Here's how the part is built. I have some questions about the finished solid (model axes, mm). Face numbers are marked on the shaded views. A direction names the side the tool comes from. Give positions to 0.01 mm unless a question says otherwise; leave off trailing zeros. Loops run counter-clockwise (first coordinate to the right, second up) from the corner with the lowest first, then second, coordinate; pieces in that order, holes last. Notation, with made-up numbers: (39.5, 20) - (56.5, 20) arc R35 ccw to (56.5, 52) - close; hole circle Ø10 at (3, 20). An arc over 180 degrees is marked (long way). Return JSON: item names as keys, results as strings. Group by question number.
(1) If we section it at A-A (x = 0): Please give me the cut outline in (y, z).
(2) If we section it at D-D (z = 157.5): Please give me the cut outline in (x, y).
(3) I need wall thicknesses on probe 1 along Z at (x, y) = (-4.5, -63); probe 2 along Z at (x, y) = (63.5, 8); probe 3 along Y at (x, z) = (-11, 166). Which ranges of each line are inside material? Lowest first, please. Write a range as [from, to].
(4) If we section it at C-C (x = 49): Please give me the cut outline in (y, z).
(5) For P1, Ø2, axis at y = -14, z = 185, coming from the -X side; P2, Ø22.5, axis at x = 12, z = 157.5, coming from the +Y side; P3, Ø9.5, axis at x = -2, z = 191, coming from the -Y side, each with a flat end and sliding along its axis, tell me the tip position at first contact or that it passes through.
(6) If we mould it in two halves opening along Y, with no side actions, what happens to the marked faces 1, 2 and 3? For each: released by +Y, released by -Y, zero draft, split by the parting line, or undercut.
(7) On a 3-axis mill with a long thin cutter (end or side, diameter ignored), from which of +Z, -Z, +X, -X, +Y, -Y can I reach the whole of each face in a straight line? I mean the marked faces 4 and 5. Say none if no direction works.
(8) If we section it at B-B (y = 0): Please give me the cut outline in (x, z).
Autodesk Inventor part; units mm, degrees
ref_plane "YZ Plane" through (0, 0, 0) normal (1, 0, 0) x (0, 1, 0)
ref_plane "XZ Plane" through (0, 0, 0) normal (0, 1, 0) x (-1, 0, 0)
ref_plane "XY Plane" through (0, 0, 0) normal (0, 0, 1) x (1, 0, 0)
sketch "Sketch1" plane through (0, 0, 0) normal (0, 0, 1) x (1, 0, 0)
  circle A0 centre (0, 0) radius 84
  dimension "d0" = 168
extrude "Extrusion1" add sketch "Sketch1" along normal blind 176
sketch "Sketch2" plane through (0, 0, 0) normal (0, 1, 0) x (-1, 0, 0)
  line L0 (84, 176) -> (-84, 176)
  circle A0 centre (0, 176) radius 28
  point P0 (0, 0)
  dimension "d3" = 56
extrude "Extrusion2" cut sketch "Sketch2" along normal mid plane 120
sketch "Sketch4" plane through (0, 0, 176) normal (0, 0, 1) x (1, 0, 0)
  line L0 (68, -28) -> (-68, -28)
  line L1 (-68, -28) -> (-68, 28)
  line L2 (-68, 28) -> (68, 28)
  line L3 (68, 28) -> (68, -28)
  line L4 (68, -28) -> (-68, 28) construction
  line L5 (-68, -28) -> (68, 28) construction
  circle A0 centre (0, 0) radius 84
  dimension "d7" = 56
  dimension "d8" = 16
extrude "Extrusion3" add sketch "Sketch4" along normal blind 24 contours L0 L1 L2 L3
sketch "Sketch5" plane through (0, 0, 200) normal (0, 0, 1) x (1, 0, 0)
  line L0 (28, -28) -> (-28, -28)
  line L1 (-12, 28) -> (12, 28)
  line L2 (12, 28) -> (12, -28)
  line L3 (12, -28) -> (-12, -28)
  line L4 (-12, -28) -> (-12, 28)
  line L5 (-12, 28) -> (12, -28) construction
  line L6 (12, 28) -> (-12, -28) construction
  point P0 (0, 0)
  dimension "d11" = 24
extrude "Extrusion4" add sketch "Sketch5" along normal blind 8
properties part number "link_1"
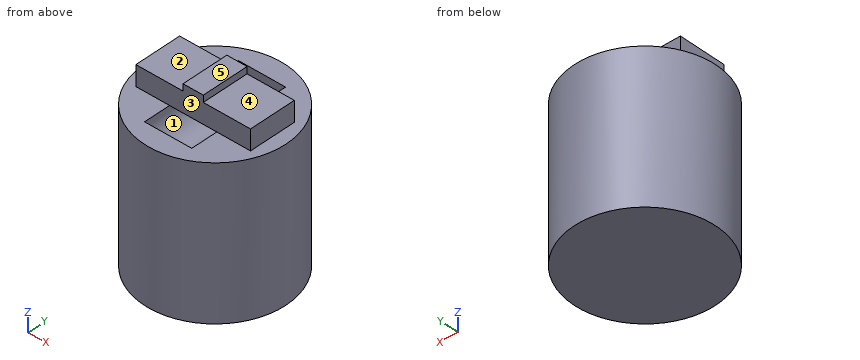
Values:
{
 "1": {"outline": "(-84, 0) - (84, 0) - (84, 176) - (60, 176) - (60, 148) - (-60, 148) - (-60, 176) - (-84, 176) - close; (-28, 176) - (28, 176) - (28, 208) - (-28, 208) - close"},
 "2": {"outline": "circle Ø168 at (0, 0); hole (-21.02, -60) - (21.02, -60) - (21.02, 60) - (-21.02, 60) - close"},
 "3": {"probe 1": "[0, 176]", "probe 2": "[0, 200]", "probe 3": "[-83.28, -60], [60, 83.28]"},
 "4": {"outline": "(-68.23, 0) - (68.23, 0) - (68.23, 176) - (28, 176) - (28, 200) - (-28, 200) - (-28, 176) - (-68.23, 176) - close"},
 "5": {"P1": "x = -68", "P2": "y = 84", "P3": "y = -28"},
 "6": {"face 1": "undercut", "face 2": "zero draft", "face 3": "released by -Y"},
 "7": {"face 4": "+Z, +X, +Y, -Y", "face 5": "+Z, +X, -X, +Y, -Y"},
 "8": {"outline": "(-84, 0) - (84, 0) - (84, 176) - (68, 176) - (68, 200) - (12, 200) - (12, 208) - (-12, 208) - (-12, 200) - (-68, 200) - (-68, 176) - (-84, 176) - close; hole (-28, 176) arc R28 ccw to (28, 176) - close"}
}
